The figure shows three views and two pictorial views of one solid part (mm, origin at its lowest corner). Answer the questions. A direction names the side the tool comes from. Round coordinates to 2 decimals unless told otherwise and drop trailing zeros. Order: outer loops, then holes, each group sorted by start corner. A loop starts at its lowest first (then second) coordinate and runs counter-clockwise, first axis right, second up.
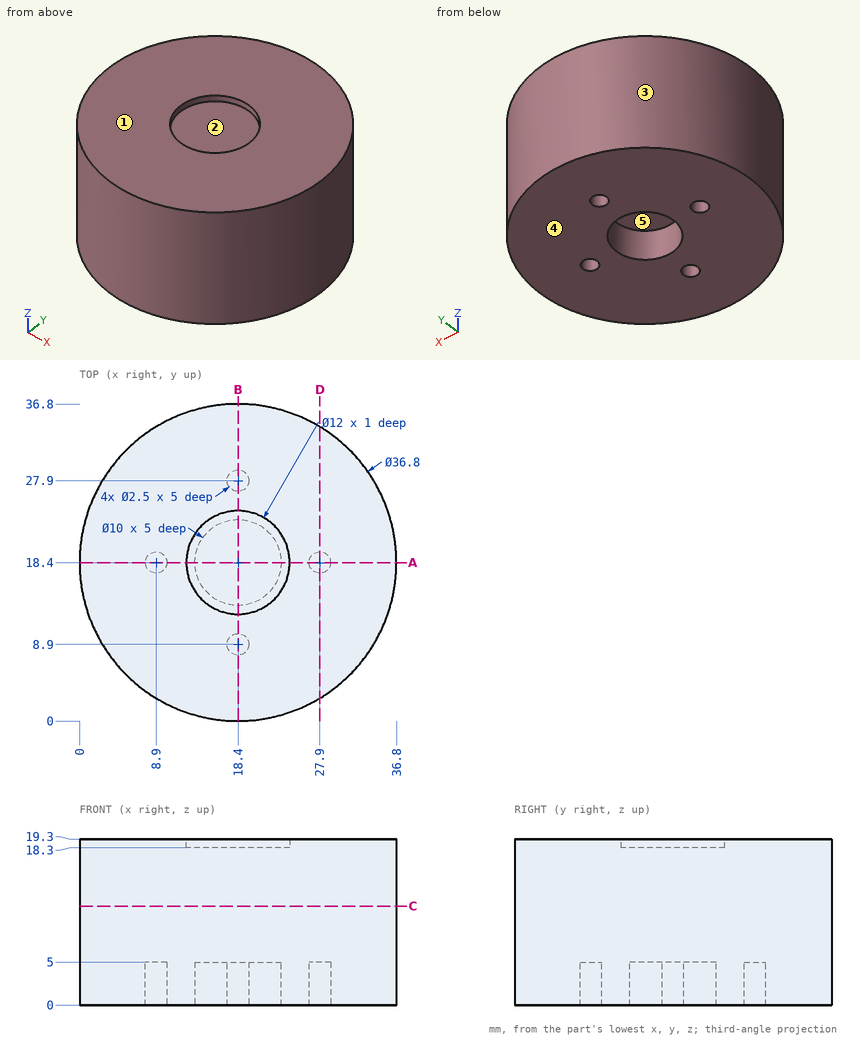
Item 1: Find section A-A (y = 18.4). Write down the section's boundary in (x, z), plus the area to 3 significant figures.
Item 2: Find section C-C (z = 11.5). Write down the section's boundary in (x, y), plus the area to 3 significant figures.
Item 3: A tool of negligible diameter and unlimited length cuts with its end or side. For the marked faces 4 and 5, from which of +Z, -Z, +X, -X, +Y, -Y can it reach the whole face along a straight path? Write none if from no direction.
Item 4: For a pull along Y with two mould halves and no side action, classify the marked faces 1, 2 and 3 as released by +Y, released by -Y, zero draft, split by the parting line, or undercut.
Item 5: Find the intervals of material crossed by line 1 along Y through (x, z) = (18.4, 2.9); line 2 along Y through (x, z) = (18.4, 18.65); line 3 along Z through (x, y) = (13, 17.5), in increasing order.
Item 6: Find section D-D (x = 27.9). Write down the section's boundary in (y, z), plus the area to 3 significant figures.
Item 7: Given pin 1 (1.2 mm diameter, centred on x = 27.5, y = 18, fed in from -Z); pin 2 (3 mm diameter, centred on x = 18.4, y = 27.9, fed in from -Z); pin 3 (8 mm diameter, centred on y = 24.5, z = 14, fed in from +X); pin 4 (3 mm diameter, centred on y = 21, z = 7, fed in from -X), each flat-ended and moving along its own axis, determine where each tip first touches the part or whether it passes through.
Model answer:
1. outline: (0, 0) - (7.65, 0) - (7.65, 5) - (10.15, 5) - (10.15, 0) - (13.4, 0) - (13.4, 5) - (23.4, 5) - (23.4, 0) - (26.65, 0) - (26.65, 5) - (29.15, 5) - (29.15, 0) - (36.8, 0) - (36.8, 19.3) - (24.4, 19.3) - (24.4, 18.3) - (12.4, 18.3) - (12.4, 19.3) - (0, 19.3) - close
1. area: 623 mm2
2. outline: circle Ø36.8 at (18.4, 18.4)
2. area: 1,060 mm2
3. face 4: -Z, +X, -X, +Y, -Y
3. face 5: -Z
4. face 1: zero draft
4. face 2: undercut
4. face 3: split by the parting line
5. line 1: y = 0 to 7.65, 10.15 to 13.4, 23.4 to 26.65, 29.15 to 36.8
5. line 2: y = 0 to 12.4, 24.4 to 36.8
5. line 3: z = 0 to 18.3
6. outline: (2.64, 0) - (17.15, 0) - (17.15, 5) - (19.65, 5) - (19.65, 0) - (34.16, 0) - (34.16, 19.3) - (2.64, 19.3) - close
6. area: 596 mm2
7. pin 1: stops at z = 5
7. pin 2: stops at z = 0
7. pin 3: stops at x = 36.68
7. pin 4: stops at x = 0.03
